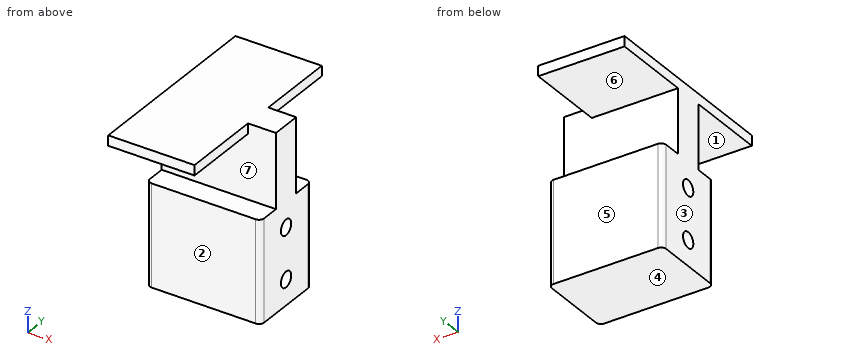
Autodesk Inventor part; units mm, degrees
ref_plane "YZ Plane" through (0, 0, 0) normal (1, 0, 0) x (0, 1, 0)
ref_plane "XZ Plane" through (0, 0, 0) normal (0, 1, 0) x (-1, 0, 0)
ref_plane "XY Plane" through (0, 0, 0) normal (0, 0, 1) x (1, 0, 0)
sketch "Sketch1" plane through (0, 0, 0) normal (1, 0, 0) x (0, 1, 0)
  circle A0 centre (0, -10) radius 3.05
  circle A1 centre (0, -30) radius 3.05
  line L0 (0, 0) -> (6, 0)
  line L1 (6, 0) -> (6, -40)
  line L2 (6, -40) -> (-6, -40)
  line L3 (-6, -40) -> (-6, 0)
  line L4 (-6, 0) -> (0, 0)
  line L5 (6, 0) -> (-6, 0)
extrude "Extrusion1" add sketch "Sketch1" along normal blind 4
sketch "Sketch2" plane through (0, -6, 0) normal (0, 0, 1) x (1, 0, 0)
  line L0 (0, 12) -> (0, 0)
  line L1 (0, 0) -> (4, 0)
  line L2 (4, 12) -> (4, 0)
  line L3 (0, 12) -> (4, 12)
  point P0 (0, 6)
extrude "Extrusion2" add sketch "Sketch2" along normal blind 29.25
sketch "Sketch3" plane through (0, -6, 29.25) normal (0, 0, 1) x (1, 0, 0)
  line L0 (0, 0) -> (0, 12)
  line L1 (0, 12) -> (0, 43.7)
  line L2 (0, 0) -> (4, 0)
  line L3 (0, 0) -> (0, -31.7)
  line L4 (0, 43.7) -> (34, 43.7)
  line L5 (0, -31.7) -> (34, -31.7)
  line L6 (34, -31.7) -> (34, 43.7)
  line L7 (0, 12) -> (0, 0)
  line L8 (0, 0) -> (4, 0)
  line L9 (4, 0) -> (4, 12)
  line L10 (4, 12) -> (0, 12)
  point P0 (0, 6)
  dimension "d12" = 31.7
  dimension "d13" = 31.7
  dimension "d14" = 34
  dimension "d15" = 34
extrude "Extrusion3" add sketch "Sketch3" against normal blind 4 contours L2 L9 L10 L1 L4 L6 L5 L3
sketch "Sketch4" plane through (4, 0, 0) normal (1, 0, 0) x (0, 0, -1)
  line L0 (-25.25, 6) -> (-25.25, -6)
  line L1 (40, -6) -> (-25.25, -6)
  line L2 (40, -6) -> (40, 6)
  line L3 (40, 6) -> (-25.25, 6)
  circle A0 centre (10, 0) radius 3.05
  circle A1 centre (30, 0) radius 3.05
  point P0 (0, 0)
extrude "Extrusion4" add sketch "Sketch4" along normal blind 41
sketch "Sketch5" plane through (34, -6, 25.25) normal (0, 0, 1) x (1, 0, 0)
  line L0 (0, 12) -> (0, 0)
  line L1 (0, 0) -> (11, 0)
  line L2 (11, 12) -> (11, 0)
  line L3 (0, 12) -> (11, 12)
  point P0 (-34, 6)
extrude "Extrusion5" add sketch "Sketch5" along normal up to surface (4 mm away)
sketch "Sketch6" plane through (0, 6, 25.25) normal (0, 1, 0) x (1, 0, 0)
  line L0 (45, 65.25) -> (45, -4)
  line L1 (45, 65.25) -> (45, 25.25)
  line L2 (45, 25.25) -> (0, 25.25)
  line L3 (0, 65.25) -> (45, 65.25)
  line L4 (0, 25.25) -> (0, 65.25)
  line L5 (0, 65.25) -> (45, 65.25)
  dimension "d23" = 40
extrude "Extrusion6" add sketch "Sketch6" along normal blind 9
fillet "Fillet2" radius 2 2 edges at (0, 15, -20) (45, 15, -20)
sketch "Sketch7" plane through (0, -6, 25.25) normal (0, -1, 0) x (1, 0, 0)
  line L0 (45, -25.25) -> (45, -65.25)
  line L1 (45, -65.25) -> (45, -25.25)
  line L2 (45, -25.25) -> (0, -25.25)
  line L3 (45, -25.25) -> (0, -25.25)
  line L4 (0, -25.25) -> (0, -65.25)
  line L5 (0, -65.25) -> (45, -65.25)
extrude "Extrusion7" add sketch "Sketch7" along normal blind 9
fillet "Fillet3" radius 2 2 edges at (45, -15, -20) (0, -15, -20)
properties part number "din_lamp_connector"
For this review, take the finished solid that the model builds, in its own axes (mm). Face numbers are marked on the shaded views. A direction names the side the tool comes from. Round coordinates to 2 decimals unless told otherwise and drop trailing zeros. Write each loop counter-clockwise with the first axis right and the second up, starting at its lowest first coordinate (ties: lowest second). Pieces come first, ordered by that corner, then holes. Notation, with made-up numbers: M 37,-7 L 82,-7 A19 cw 82,19 Z; hole C 48,14 d9. An arc over 180 degrees is marked long. One line per item, written item: value. Start each with the question number.
(1) Wall thickness on line 1 (Z direction, x = 17, y = 0); line 2 (Y direction, x = 30, z = -30); line 3 (Y direction, x = 17, z = 18.5): over which ranges is each line inside the solid? List them lowest first.
(2) We need section C-C (z = -22). Give the boundary of the cut face in (x, y), and give its area (3 significant figures).
(3) We need section A-A (x = 9). Give the boundary of the cut face in (y, z).
(4) We need section B-B (y = -11.5). Give the boundary of the cut face in (x, z), and give its area (3 significant figures).
(5) We need section D-D (y = -21). Give the boundary of the cut face in (x, z).
(6) Machinability: for the marked faces 1, 2 and 3, which of the approach directions +Z, -Z, +X, -X, +Y, -Y give a long, thin tool a straight path to every point of the face, cutting with its end or side? Answer none if there is none.
(7) The part is to be moulded in two halves that separate along Z. For the marked faces 4, 5, 6 and 7, say which applies: released by +Z, released by -Z, zero draft, split by the parting line, or undercut.
(8) Insertion check: pin 1 (1.2 mm diameter, centred on y = 25.5, z = 26.5, fed in from +X); pin 2 (23.5 mm diameter, centred on x = 23.5, z = 8.5, fed in from +Y); pin 3 (6 mm diameter, centred on x = 8, z = 10.5, fed in from -Y). Each pin has a flat end and moves straight along its axis. Give the tip position at first contact, or say it passes through.
Result:
1. line 1: -40 to -33.05, -26.95 to -13.05, -6.95 to 29.25
1. line 2: -15 to -3.05, 3.05 to 15
1. line 3: -6 to 6
2. outline: M 0,-13 A2 ccw 2,-15 L 43,-15 A2 ccw 45,-13 L 45,13 A2 ccw 43,15 L 2,15 A2 ccw 0,13 Z
2. area: 1,350 mm²
3. outline: M -37.7,25.25 L -6,25.25 L -6,0 L -15,0 L -15,-40 L 15,-40 L 15,0 L 6,0 L 6,25.25 L 37.7,25.25 L 37.7,29.25 L -37.7,29.25 Z; hole C 0,-30 d6.1; hole C 0,-10 d6.1
4. outline: M 0,-40 L 45,-40 L 45,0 L 0,0 Z; M 0,25.25 L 34,25.25 L 34,29.25 L 0,29.25 Z
4. area: 1,940 mm²
5. outline: M 0,25.25 L 34,25.25 L 34,29.25 L 0,29.25 Z
6. face 1: +X, -X, -Y
6. face 2: -Z, +X, -X, -Y
6. face 3: +Z, -Z, -X, +Y, -Y
7. face 4: released by -Z
7. face 5: zero draft
7. face 6: undercut
7. face 7: undercut
8. pin 1: x = 34
8. pin 2: y = 15
8. pin 3: y = -6
